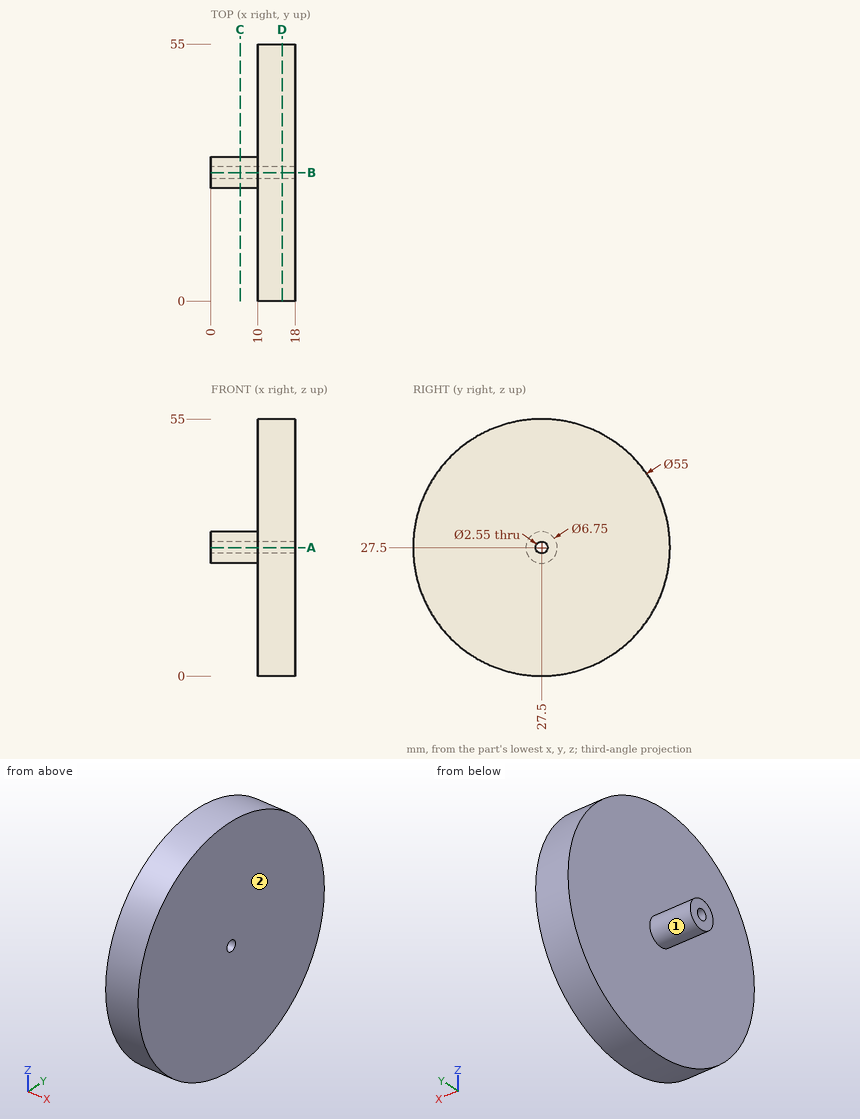
Input: dimensioned drawing with shaded views. Units: mm. Origin: part minimum x, y, z. A direction names the side the tool comes from. Give positions to 0.01 mm unless a question says otherwise; leave off trailing zeros. Order: outer loops, then holes, each group sorted by start corner. A loop starts at its lowest first (then second) coordinate and runs counter-clockwise, first axis right, second up. Notation, with made-up numbers: (2.25, -19) -> (41.25, -19) arc R7 ccw to (41.25, -6) -> close; hole circle Ø10 at (79, 15.5). An arc over 180 degrees is marked (long way). Write item = value, one per line.
Item 1: Ray query, probe 1 along Z at (x, y) = (8.75, 27.5) (3 decimals); probe 2 along X at (y, z) = (44.5, 12); probe 3 along Z at (x, y) = (10.5, 27.5) (3 decimals). Return the intervals inside material, ascending.
Check result:
probe_1 = 24.125 to 26.225, 28.775 to 30.875
probe_2 = 10 to 18
probe_3 = 0 to 26.225, 28.775 to 55
Item 2: Section query C-C (x = 6.25). Output: boundary loops of the cut face in (y, z) (3 decimals).
Check result:
outline = circle Ø6.75 at (27.5, 27.5); hole circle Ø2.55 at (27.5, 27.5)
Item 3: Contact query for flat-ended pins moving along their axis: pin 1 (5 mm diameter, centred on x = 12.5, y = 36.5, fed in from +Z); pin 2 (4 mm diameter, centred on x = 9, y = 7, fed in from -Z); pin 3 (5 mm diameter, centred on x = 12, y = 41.5, fed in from +Z); pin 4 (4 mm diameter, centred on x = 6.5, y = 15, fed in from -Z). Output: stop coordinate, or through.
Check result:
pin_1 = 54.22
pin_2 = 7.4
pin_3 = 52.48
pin_4 = through
Item 4: Set-up query: the marked faces 1 and 2. Return all of +Z, -Z, +X, -X, +Y, -Y with unobstructed straight access to the full face (end or side cutting, diameter ignored); none if empty.
Check result:
face_1 = -X
face_2 = +Z, -Z, +X, +Y, -Y
Item 5: Section query D-D (x = 15.25). Output: boundary loops of the cut face in (y, z) (3 decimals), then the cut area to 3 significant figures.
Check result:
outline = circle Ø55 at (27.5, 27.5); hole circle Ø2.55 at (27.5, 27.5)
area = 2,370 mm²
Item 6: Section query A-A (z = 27.5). Output: boundary loops of the cut face in (x, y) (3 decimals).
Check result:
outline = (0, 24.125) -> (10, 24.125) -> (10, 0) -> (18, 0) -> (18, 26.225) -> (0, 26.225) -> close; (0, 28.775) -> (18, 28.775) -> (18, 55) -> (10, 55) -> (10, 30.875) -> (0, 30.875) -> close
